Autodesk Inventor part; units mm, degrees
ref_plane "YZ Plane" through (0, 0, 0) normal (1, 0, 0) x (0, 1, 0)
ref_plane "XZ Plane" through (0, 0, 0) normal (0, 1, 0) x (-1, 0, 0)
ref_plane "XY Plane" through (0, 0, 0) normal (0, 0, 1) x (1, 0, 0)
sketch "Esboço2" plane through (0, 0, 0) normal (0, 0, 1) x (1, 0, 0)
  circle A0 centre (0, 0) radius 2.5
  line L0 (10, 10) -> (10, -10) construction
  line L1 (10, 3.1) -> (10, -3.1) construction
  line L2 (4, 3.1) -> (4, -3.1) construction
  line L3 (0, 0) -> (2.5, 0) construction
  line L4 (10, 10) -> (10, 3.1) construction
  line L5 (10, 3.1) -> (8, 3.1) construction
  line L6 (8, 3.1) -> (8, 6.8) construction
  line L7 (8, 6.8) -> (4, 3.1) construction
  line L8 (10, -3.1) -> (10, -10) construction
  line L9 (8, -3.1) -> (10, -3.1) construction
  line L10 (8, -3.1) -> (8, -6.8) construction
  line L11 (8, -6.8) -> (4, -3.1) construction
  line L12 (10, 3.1) -> (9.5, 3.1) construction
  line L13 (9.5, 3.1) -> (9.5, 3.6)
  line L14 (9.5, 3.6) -> (10, 3.6)
  line L15 (10, 3.6) -> (10, 3.1) construction
  line L16 (10, 10) -> (10, 3.6) construction
  line L17 (9.5, 3.1) -> (8, 3.1)
  line L18 (10, -3.1) -> (9.5, -3.1) construction
  line L19 (9.5, -3.1) -> (9.5, -3.6)
  line L20 (9.5, -3.6) -> (10, -3.6)
  line L21 (10, -3.6) -> (10, -3.1) construction
  line L22 (10, -3.6) -> (10, -10) construction
  line L23 (8, -3.1) -> (9.5, -3.1)
  line L24 (0, 0) -> (0, -2.5) construction
  line L25 (0, 2.5) -> (0, 0) construction
  arc A1 (10, 9.5) -> (9.5, 10) centre (9.5, 9.5) ccw
  line L26 (10, 9.5) -> (10, 3.6)
  line L27 (-10, 10) -> (10, 10) construction
  line L28 (-10, 10) -> (-10, -10) construction
  line L29 (0, 0) -> (-10, 10) construction
  line L30 (-2.5, 0) -> (0, 0) construction
  arc A2 (8, 5.6564) -> (7.1605, 6.0234) centre (7.5, 5.6564) ccw
  line L31 (8, 5.6564) -> (8, 3.1)
  arc A3 (7.1605, -6.0234) -> (8, -5.6564) centre (7.5, -5.6564) ccw
  arc A4 (4.1605, 3.2484) -> (4, 2.8814) centre (4.5, 2.8814) ccw
  arc A5 (4, -2.8814) -> (4.1605, -3.2484) centre (4.5, -2.8814) ccw
  line L32 (4, 2.8814) -> (4, -2.8814)
  line L33 (4.1605, -3.2484) -> (7.1605, -6.0234)
  line L34 (4.1605, 3.2484) -> (7.1605, 6.0234)
  line L35 (8, -3.1) -> (8, -5.6564)
  arc A6 (9.5, -10) -> (10, -9.5) centre (9.5, -9.5) ccw
  line L36 (10, -3.6) -> (10, -9.5)
  arc A7 (9.5, 10) -> (-10, -9.5) centre (9.5, -9.5) ccw
  arc A8 (-10, -9.5) -> (-9.5, -10) centre (-9.5, -9.5) ccw
  line L37 (-3.1, 4.3108) -> (3.1, 4.3108) construction
  line L38 (3.1, 4.3108) -> (8, 8.8433) construction
  arc A9 (6.8948, 7.821) -> (6.4827, 8.6828) centre (6.5553, 8.1881) ccw
  arc A10 (2.9042, 4.3108) -> (3.2437, 4.4438) centre (2.9042, 4.8108) ccw
  arc A11 (8, 8.8433) -> (-3.1, 4.3108) centre (9.2294, -10.0255) ccw construction
  arc A12 (-1.9647, 5.2138) -> (-1.6687, 4.3108) centre (-1.6687, 4.8108) ccw
  line L39 (-1.6687, 4.3108) -> (2.9042, 4.3108)
  arc A13 (6.4827, 8.6828) -> (-1.9647, 5.2138) centre (9.2294, -10.0255) ccw
  line L40 (3.2437, 4.4438) -> (6.8948, 7.821)
  line L41 (-6.8, -8) -> (-3.1, -8) construction
  line L42 (-10, -10) -> (10, -10) construction
  line L43 (-3.1, -10) -> (3.1, -10) construction
  line L44 (-10, -10) -> (-3.1, -10) construction
  line L45 (-9.5, -10) -> (-3.1, -10) construction
  line L46 (-3.1, -8) -> (-3.1, -10) construction
  line L47 (3.1, -10) -> (10, -10) construction
  line L48 (3.1, -8) -> (3.1, -10) construction
  line L49 (3.1, -8) -> (7.0883, -8) construction
  line L50 (3.1, -10) -> (9.5, -10) construction
  line L51 (2.764, -4) -> (7.0883, -8) construction
  line L52 (-2.764, -4) -> (2.764, -4) construction
  line L53 (-6.8, -8) -> (-2.764, -4) construction
  arc A14 (-5.9372, -7.1449) -> (-5.5852, -8) centre (-5.5852, -7.5) ccw
  arc A15 (-2.5582, -4) -> (-2.9101, -4.1449) centre (-2.5582, -4.5) ccw
  arc A16 (2.9077, -4.133) -> (2.5682, -4) centre (2.5682, -4.5) ccw
  arc A17 (5.8114, -8) -> (6.151, -7.133) centre (5.8114, -7.5) ccw
  line L54 (-3.1, -10) -> (-3.6, -10) construction
  line L55 (-3.6, -10) -> (-3.6, -9.5)
  line L56 (-3.6, -9.5) -> (-3.1, -9.5)
  line L57 (-3.1, -9.5) -> (-3.1, -10) construction
  line L58 (-9.5, -10) -> (-3.6, -10)
  line L59 (-3.1, -9.5) -> (-3.1, -8)
  line L60 (-2.9101, -4.1449) -> (-5.9372, -7.1449)
  line L61 (-2.5582, -4) -> (2.5682, -4)
  line L62 (6.151, -7.133) -> (2.9077, -4.133)
  line L63 (3.1, -8) -> (5.8114, -8)
  line L64 (-5.5852, -8) -> (-3.1, -8)
  line L65 (3.1, -10) -> (3.6, -10) construction
  line L66 (3.6, -10) -> (3.6, -9.5)
  line L67 (3.6, -9.5) -> (3.1, -9.5)
  line L68 (3.1, -9.5) -> (3.1, -10) construction
  line L69 (3.6, -10) -> (9.5, -10)
  line L70 (3.1, -8) -> (3.1, -9.5)
  line L71 (-8.9309, -8) -> (-4, -3.1131) construction
  line L72 (-4, -3.1131) -> (-4, 2.889) construction
  arc A18 (-4, 2.889) -> (-8.9309, -8) centre (9.8766, -9.9556) ccw construction
  arc A19 (-8.7144, -6.503) -> (-7.8708, -6.9494) centre (-8.2228, -6.5943) ccw
  arc A20 (-4, 1.5422) -> (-4.8905, 1.8545) centre (-4.5, 1.5422) ccw
  arc A21 (-4.148, -3.2598) -> (-4, -2.9047) centre (-4.5, -2.9047) ccw
  arc A22 (-4.8863, 1.8598) -> (-8.7144, -6.503) centre (9.8766, -9.9556) ccw
  line L73 (-4, 1.5422) -> (-4, -2.9047)
  line L74 (-4.148, -3.2598) -> (-7.8708, -6.9494)
  point P0 (10, 0)
  point P1 (10, 0)
  point P2 (4, 0)
  point P3 (0, 4.3108)
  point P4 (0, -10)
  point P5 (0, -10)
  point P6 (10, 6.8)
  point P7 (8, -4.3782)
  point P8 (0, -4)
  point P9 (-4.8905, 1.8545)
  dimension "d6" = 5
  dimension "d7" = 20
  dimension "d8" = 10
  dimension "d9" = 6.2
  dimension "d11" = 6
  dimension "d17" = 2
  dimension "d22" = 0.5
  dimension "d24" = 0.5
  dimension "d65" = 1.5
  dimension "d67" = 1.5
  dimension "d69" = 1.5
  dimension "d70" = 1.5
  dimension "d72" = 1.5
extrude "Extrusão1" add sketch "Esboço2" along normal mid plane 2000
properties part number "Perfil 20×20 R90 2 rasgos" material "Ouro"
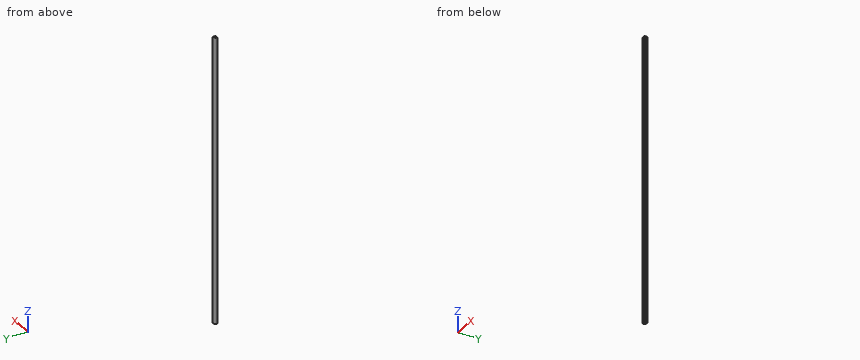
Build history of the part. All positions in model axes, mm. Coordinates: 2 decimals unless noted, no trailing zeros. Use CSV: the item, a comma, the result in double quotes. Start each with the question number.
Q1. Flat gauge pins, fed straight in: pin 1 Ø2.5 at (x, z) = (-4, -323) entering from +Y; pin 2 Ø1.5 at (x, z) = (-1, -22.5) entering from -Y; pin 3 Ø3 at (y, z) = (5, -328) entering from -X. Where does each tip first touch, or does it go through?
Q2. Drill centre lines: probe 1 along Y at (x, z) = (-4.75, 502.5); probe 2 along Y at (x, z) = (5.25, -278.5); probe 3 along Y at (x, z) = (0, 148). Where is each one in solid material? Low to high.
Q3. Cut at A-A, the plane z = -121. State how many separate pieces and enclosed holes the cut face has, then the cut area to 3 significant figures.
Checked values:
1,pin 1,"stops at y = 5.67"
1,pin 2,"stops at y = -4"
1,pin 3,"stops at x = -5.03"
2,probe 1,"y = -10 to -8, -5.97 to -3.86, 1.98 to 3.81"
2,probe 2,"y = -10 to -8, -6.3 to -4.26, 4.26 to 6.3, 8.46 to 9.53"
2,probe 3,"y = -4 to -2.5, 2.5 to 4.31, 6.48 to 7.53"
3,separate pieces,"1"
3,enclosed holes,"3"
3,area,"153 mm²"
